The model under review builds one solid part; all positions refer to its coordinate system, in mm. A direction names the side the tool comes from. Give positions to 0.01 mm unless a question says otherwise; leave off trailing zeros. Order: outer loops, then holes, each group sorted by start corner. A loop starts at its lowest first (then second) coordinate and runs counter-clockwise, first axis right, second up. Notation, with made-up numbers: (73, -28) -> (127, -28) arc R16 cw to (127, -3) -> close; hole circle Ø4 at (-13.75, -35). An arc over 180 degrees is marked (long way). Use one line per item in the form item = value.
```python
from build123d import *

# Parameters (mm, degrees)
BOSS_EXTRUDE1_DEPTH        = 20.32
F_8_0_199_DIAMETER_HOLE1_D = 4.191
CUT_EXTRUDE1_DEPTH         = 262.594137913
CUT_EXTRUDE1_DEPTH_BACK    = 262.594137913
SKETCH4_R                  = 2.0955


with BuildPart() as part:
    # Sketch1 → Boss-Extrude1 (new body)
    with BuildSketch(Plane(origin=(0, 0, 0), x_dir=(0, 0, -1), z_dir=(1, 0, 0))):
        with BuildLine():
            Line((-96.165603327, -175.75792688), (-116.485603327, -175.75792688))
            Line((-116.485603327, -175.75792688), (-116.485603327, 27.44207312))
            ThreePointArc((-116.485603327, 27.44207312), (-134.944175413, 48.803773877), (-158.757234566, 33.6387036))
            ThreePointArc((-158.757234566, 33.6387036), (-167.922977729, 20.553260194), (-183.088565435, 15.528857106))
            Line((-183.088565435, 15.528857106), (-192.685603327, 15.528857106))
            Line((-192.685603327, 15.528857106), (-188.14698461, 34.403768669))
            Line((-188.14698461, 34.403768669), (-169.26182214, 55.43971331))
            ThreePointArc((-169.26182214, 55.43971331), (-123.085045139, 66.579411625), (-96.165603327, 27.44207312))
            Line((-96.165603327, 27.44207312), (-96.165603327, -175.75792688))
        make_face()
    extrude(amount=BOSS_EXTRUDE1_DEPTH)

    # #8 (0.199) Diameter Hole1 (through all)
    with Locations(Plane.XY.offset(116.485603327)):
        with Locations((10.16, -89.697235998), (10.16, -115.097235998), (10.16, -140.497235998), (10.16, -165.897235998), (10.16, -191.297235998)):
            Hole(F_8_0_199_DIAMETER_HOLE1_D / 2)

    # Sketch4 → Cut-Extrude1 (cut, two sides: drawn at the far end of the back side and taken through both)
    with BuildSketch(Plane(origin=(20.32, 0, 0), x_dir=(0, 0, -1), z_dir=(1, 0, 0)).offset(-CUT_EXTRUDE1_DEPTH_BACK)):
        with Locations((-175.949281774, 28.226562255)):
            Circle(SKETCH4_R)
        with Locations((-159.099223615, 50.683912634)):
            Circle(SKETCH4_R)
        with Locations((-112.3119526, 45.871678806)):
            Circle(SKETCH4_R)
        with Locations((-105.851443143, 20.865071419)):
            Circle(SKETCH4_R)
    extrude(amount=CUT_EXTRUDE1_DEPTH + CUT_EXTRUDE1_DEPTH_BACK, mode=Mode.SUBTRACT)


solid = part.part
```
1. Add section B-B on z = 127. Give the boundary of the cut face in (x, y).
Values:
outline = (0, 45.97) -> (20.32, 45.97) -> (20.32, 67.86) -> (0, 67.86) -> close
2. For L1, parallel to Z at x = 4, y = -121; L2, parallel to Y at x = 5.25, z = 105.5; L3, parallel to Y at x = 8, z = 113.5, list the stretches that pass through material, from the lowest coordinate up.
Values:
L1 = 96.17 to 116.49
L2 = -175.76 to 18.8, 22.93 to 53.81
L3 = -175.76 to 44.15, 47.6 to 61.39
3. Add section C-C on y = -59. Give the boundary of the cut face in (x, z).
Values:
outline = (0, 96.17) -> (20.32, 96.17) -> (20.32, 116.49) -> (0, 116.49) -> close
4. Tool access review of faces 4 (the face through (10, 15.529, 188)), 5 (the face through (10.02, 20.69, 167.74)), 6 (the face through (10, -73, 96.166)): name each direction out of +Z, -Z, +X, -X, +Y, -Y from which nothing blocks a thin tool from reaching the whole face with its end or side.
Values:
face_4 = +Z, +X, -X, -Y
face_5 = +X, -X, -Y
face_6 = -Z, +X, -X, +Y, -Y
5. The part is to be moulded in two halves that separate along X. For faces 1 (the face through (10.614, -142.543, 106.183)), 2 (the face through (0, -25, 116)), 3 (the face through (10, -175.758, 106)), say which applies: +X half, -X half, draft (parallel to the pull), parting line (faces both ways), or undercut.
Values:
face_1 = undercut
face_2 = -X half
face_3 = draft
6. For pin 1 Ø8 at (x, z) = (12.5, 144) entering from +Y; pin 2 Ø8 at (x, z) = (5, 143) entering from -Y; pin 3 Ø10 at (x, z) = (3.5, 165.5) entering from +Y, all flat-tipped, find the tip position at first contact; note any pin that passes through.
Values:
pin_1 = 69.31
pin_2 = 47.1
pin_3 = 62.85
7. Add section A-A on x = 16. Give the boundary of the cut face in (y, z), then the cut area to 3 significant figures.
Values:
outline = (-175.76, 96.17) -> (27.44, 96.17) arc R41.91 ccw to (55.44, 169.26) -> (34.4, 188.15) -> (15.53, 192.69) -> (15.53, 183.09) arc R25.4 ccw to (33.64, 158.76) arc R21.59 cw to (27.44, 116.49) -> (-175.76, 116.49) -> close; hole circle Ø4.19 at (20.87, 105.85); hole circle Ø4.19 at (28.23, 175.95); hole circle Ø4.19 at (45.87, 112.31); hole circle Ø4.19 at (50.68, 159.1)
area = 6,510 mm^2
